CAD build for the part. Positions are in the model's coordinates, mm. A direction names the side the tool comes from. Coordinates: 2 decimals unless noted, no trailing zeros. Write each loop counter-clockwise with the first axis right and the second up, starting at its lowest first coordinate (ties: lowest second). Pieces come first, ordered by that corner, then holes. Notation, with made-up numbers: (62, 69) - (105, 69) arc R18 ccw to (105, 85) - close; hole circle Ø8 at (19, 24). An arc over 180 degrees is marked (long way). One line per question, with ' | ' between items. Start each with the question number.
1. Probe line 1 (Y direction, x = 41, z = 0); line 2 (Y direction, x = 8, z = 0); line 3 (X direction, y = -4, z = 11). List the from-to ranges inside material, lowest first.
2. Two-plate mould, pull along Z, no slides. Class faces 1 (the flat face through (2, 11, 4)), 2 (the cylindrical face through (1.014, 17.084, -3.794)), 3 (the cylindrical face through (43.02, -1.88, 5.96)): +Z half, -Z half, draft (parallel to the pull), parting line (faces both ways), or undercut.
3. Band-saw the part on B-B, the plane x = 36. Write the cut outline in (y, z), then the cut area to 3 significant figures.
4. Flat gauge pins, fed straight in: P1, Ø1.5, axis at y = 3, z = 5.5, coming from the -X side; P2, Ø10, axis at x = 7.5, y = -2, coming from the -Z side; P3, Ø1.9, axis at y = 14.5, z = 0, coming from the -X side; P4, Ø2, axis at x = 48.5, y = -3, coming from the +Z side. Where does each tip first touch, or does it go through?
5. Band-saw the part on C-C, the plane z = 0. Give the number of separate pieces and of enclosed holes in the cut face, then the cut area to 3 significant figures.
6. Band-saw the part on D-D, the plane y = 14.5. Write the cut outline in (x, z).
7. Which spindle directions (+Z, -Z, +X, -X, +Y, -Y) get a long thin tool onto all of the face, cutting with end or side? Do faces 4 (the flat face through (26.5, 1.87, 6.13)), 5 (the cylindrical face through (0.986, 16.086, -0.208)), 6 (the cylindrical face through (52.6, 7.81, -1.73)). Say none if no direction does.
from build123d import *

# Parameters (mm, degrees)
CHAMFER_1_SIZE      = 1.5
CHAMFER_2_SIZE      = 1
CHAMFER_3_SIZE      = 1
CHAMFER_4_SIZE      = 0.5
SKETCH_2_R          = 1.6
CUT_EXTRUDE_1_DEPTH = 10


with BuildPart() as part:
    # Эскиз1 → Повернуть1 (revolve)
    with BuildSketch(Plane.XY, mode=Mode.PRIVATE) as revolve_1_sk:
        Polygon((26.5, 6.25), (26.5, 9), (0, 9), (0, 17.5), (2, 17.5), (2, 11.5), (29.5, 11.5), (29.5, 8.5), (45.5, 8.5), (45.5, 8), (60.5, 8), (60.5, 6.25), align=None)
    revolve(revolve_1_sk.sketch.rotate(Axis((0, 0, 0), (1, 0, 0)), 90), axis=Axis((0, 0, 0), (1, 0, 0)))

    # Фаска1
    chamfer_1_edges = [part.edges().sort_by_distance(p)[0] for p in [
        (29.5, 0, -11.5),
    ]]
    chamfer(chamfer_1_edges, length=CHAMFER_1_SIZE)

    # Фаска2
    chamfer_2_edges = [part.edges().sort_by_distance(p)[0] for p in [
        (0, 0, -9),
    ]]
    chamfer(chamfer_2_edges, length=CHAMFER_2_SIZE)

    # Фаска3
    chamfer_3_edges = [part.edges().sort_by_distance(p)[0] for p in [
        (60.5, 0, -8),
    ]]
    chamfer(chamfer_3_edges, length=CHAMFER_3_SIZE)

    # Фаска4
    chamfer_4_edges = [part.edges().sort_by_distance(p)[0] for p in [
        (45.5, 0, -8.5),
        (60.5, 0, -6.25),
    ]]
    chamfer(chamfer_4_edges, length=CHAMFER_4_SIZE - 0.0001)  # a hair under: the kernel refuses the full size

    # Эскиз2 → Вырез-Вытянуть1 (cut)
    with BuildSketch(Plane.ZY):
        with Locations((0, 14.5)):
            Circle(SKETCH_2_R)
        with Locations((12.557368355, -7.25)):
            Circle(SKETCH_2_R)
        with Locations((-12.557368355, -7.25)):
            Circle(SKETCH_2_R)
    extrude(amount=-CUT_EXTRUDE_1_DEPTH, mode=Mode.SUBTRACT)


solid = part.part
Filled in:
1) line 1: y = -8.5 to -6.25, 6.25 to 8.5 | line 2: y = -11.5 to -9, 9 to 11.5 | line 3: x = 0 to 2
2) face 1: draft | face 2: parting line | face 3: undercut
3) outline: circle Ø17 at (0, 0); hole circle Ø12.5 at (0, 0) | area: 104 mm²
4) P1: stops at x = 26.5 | P2: stops at z = -11.5 | P3: passes through | P4: stops at z = 7.75
5) separate pieces: 3 | enclosed holes: 0 | area: 301 mm²
6) outline: (0, -9.8) - (2, -9.8) - (2, -1.6) - (0, -1.6) - close; (0, 1.6) - (2, 1.6) - (2, 9.8) - (0, 9.8) - close
7) face 4: -X | face 5: +X, -X | face 6: +X
